Geometry: final body of the model. Coordinates: model frame, mm. A direction names the side the tool comes from. Give positions to 0.01 mm unless a question says otherwise; leave off trailing zeros. Write each loop counter-clockwise with the first axis right and the second up, starting at its lowest first coordinate (ties: lowest second). Pieces come first, ordered by that corner, then holes. Notation, with made-up numbers: (30.5, 53.25) -> (63.5, 53.25) arc R15 cw to (63.5, 73.25) -> close; hole circle Ø7 at (30.25, 85). An arc over 180 degrees is marked (long way). Use CSV: the item, a comma, the result in double quotes. Start each with the question number.
1) Material intervals for line 1 (Z direction, x = -9.5, y = -1.7); line 2 (X direction, y = 0.25, z = -103.5); line 3 (X direction, y = -1.7, z = -16.75), sorted ascending. Write a range as [from, to].
2) Set-up query: faces 4 (the face through (9, 0, 0)), 5 (the face through (36.5, 1, -25)), 6 (the face through (88, 0, -46)). Return all of +Z, -Z, +X, -X, +Y, -Y with unobstructed straight access to the full face (end or side cutting, diameter ignored); none if empty.
3) Section A-A (x = 76.5). Output: boundary loops of the cut face in (y, z).
4) Draft query along X for faces 1 (the face through (12, -0.5, -7.3)), 2 (the face through (17.9, -3.5, -74.6)), 3 (the face through (15, 0, -68)). Return one class per face: pulls with the +X half, pulls with the -X half, needs draft (parallel to the pull), parting line crosses it, or undercut.
5) Section B-B (y = -1.45). Count the separate pieces of the cut face and the enclosed holes in it, plus the area to 3 significant figures.
6) Contact query for flat-ended pins moving along their axis: P1, Ø1.8, axis at x = 41, y = -2.5, coming from the -Z side; P2, Ø0.8, axis at y = 0.5, z = -1.5, coming from the -X side; P3, Ø2.5, axis at x = 34, y = -2.5, coming from the +Z side. Output: stop coordinate, or through.
```python
from build123d import *

# Parameters (mm, degrees)
SKETCH2_W                      = 14
SKETCH2_H                      = 14
BOSS_EXTRUDE1_DEPTH            = 1.5
SKETCH3_R                      = 7.5
SKETCH3_R_2                    = 4.250000483
SKETCH3_R_3                    = 4.259363822
SKETCH3_W                      = 5
SKETCH3_H                      = 5
SKETCH3_W_2                    = 29.940596835
SKETCH3_W_3                    = 6
SKETCH3_W_4                    = 15
SKETCH3_H_2                    = 15
SKETCH3_W_5                    = 2.885686077
SKETCH3_H_3                    = 6.92
SKETCH3_W_6                    = 48.043350903
SKETCH3_H_4                    = 3
BOSS_EXTRUDE2_DEPTH            = 3.5
M3_CLEARANCE_HOLE1_D           = 3.6
M3_CLEARANCE_HOLE1_CSINK_D     = 3.65
M3_CLEARANCE_HOLE1_CSINK_ANGLE = 90


with BuildPart() as part:
    # Sketch2 → Boss-Extrude1 (new body)
    with BuildSketch(Plane(origin=(0, 0, 0), x_dir=(1, 0, 0), z_dir=(0, 1, 0))):
        Polygon((90.5, 34), (90.5, 88.92), (105.066, 88.92), (105.066, 112.92), (34.566, 112.92), (34.566, 101.999439424), (12.680313923, 101.999439424), (12.680313923, 95.731483365), (-40.408317869, 95.731483365), (-44.678770934, 85.421697657), (-65.29834235, 85.421697657), (-69.197497471, 76.008304483), (-102.403943224, 76.008304483), (-102.403943224, 52.008304483), (-53.463346389, 52.008304483), (-12, 34.833624067), (-12, -12), (12, -12), (12, 20), (36.5, 20), (36.5, 34), align=None)
        with Locations((-90.403943224, 64.008304483)):
            Rectangle(SKETCH2_W, SKETCH2_H, mode=Mode.SUBTRACT)
        Polygon((-67.315017213, 67.487384202), (-61.95744916, 80.421697657), (-49.023135705, 75.064129604), (-54.380703758, 62.129816149), align=None, mode=Mode.SUBTRACT)
        with Locations((46.566, 100.92)):
            Rectangle(SKETCH2_W, SKETCH2_H, mode=Mode.SUBTRACT)
        Polygon((-31.423230611, 67.774010218), (-44.357544066, 73.131578271), (-49.715112119, 60.197264816), (-36.780798664, 54.839696762), align=None, mode=Mode.SUBTRACT)
        with Locations((-0.524094275, 75.65587615)):
            Rectangle(SKETCH2_W, SKETCH2_H, mode=Mode.SUBTRACT)
        with Locations((24.680313923, 89.999439424)):
            Rectangle(SKETCH2_W, SKETCH2_H, mode=Mode.SUBTRACT)
        with Locations((24.5, 61)):
            Rectangle(SKETCH2_W, SKETCH2_H, mode=Mode.SUBTRACT)
        with Locations((24.5, 32)):
            Rectangle(SKETCH2_W, SKETCH2_H, mode=Mode.SUBTRACT)
        with Locations((49.5, 46)):
            Rectangle(SKETCH2_W, SKETCH2_H, mode=Mode.SUBTRACT)
        with Locations((49.5, 75)):
            Rectangle(SKETCH2_W, SKETCH2_H, mode=Mode.SUBTRACT)
        with Locations((78.5, 75)):
            Rectangle(SKETCH2_W, SKETCH2_H, mode=Mode.SUBTRACT)
        with Locations((78.5, 46)):
            Rectangle(SKETCH2_W, SKETCH2_H, mode=Mode.SUBTRACT)
        Rectangle(SKETCH2_W, SKETCH2_H, mode=Mode.SUBTRACT)
        Polygon((-33.645940754, 49.211627299), (-20.711627299, 43.854059246), (-15.354059246, 56.788372701), (-28.288372701, 62.145940754), align=None, mode=Mode.SUBTRACT)
        Polygon((-42.424992732, 77.79716991), (-37.067424679, 90.731483365), (-24.133111224, 85.373915312), (-29.490679277, 72.439601857), align=None, mode=Mode.SUBTRACT)
        with Locations((62.066, 100.92)):
            Rectangle(SKETCH2_W, SKETCH2_H, mode=Mode.SUBTRACT)
        with Locations((77.566, 100.92)):
            Rectangle(SKETCH2_W, SKETCH2_H, mode=Mode.SUBTRACT)
        with Locations((93.066, 100.92)):
            Rectangle(SKETCH2_W, SKETCH2_H, mode=Mode.SUBTRACT)
    extrude(amount=BOSS_EXTRUDE1_DEPTH)

    # Sketch3 → Boss-Extrude2 (add)
    with BuildSketch(Plane.XZ):
        with Locations(Location((-0.403943224, -53.000000483, 0), (0, 0, 90))):
            Circle(SKETCH3_R)
        with Locations(Location((-0.903943224, -16.750000483, 0), (0, 0, 90))):
            Circle(SKETCH3_R_2)
        with Locations(Location((41.096056776, -60.500000483, 0), (0, 0, 90))):
            Circle(SKETCH3_R_3)
        with Locations(Location((16.096056776, -75.500000483, 0), (0, 0, 90))):
            Circle(SKETCH3_R_3)
        Polygon((-20.711627299, -43.854059246), (-22.625044461, -39.234661583), (-12, -34.833624067), (-12, -7), (-7, -7), (-7, -40.245585068), (-12, -40.245585068), align=None)
        with Locations((37.066, -110.42)):
            Rectangle(SKETCH3_W, SKETCH3_H)
        with Locations((102.566, -110.42)):
            Rectangle(SKETCH3_W, SKETCH3_H)
        with Locations((102.566, -91.42)):
            Rectangle(SKETCH3_W, SKETCH3_H)
        with Locations((88, -36.5)):
            Rectangle(SKETCH3_W, SKETCH3_H)
        with Locations((34, -22.5)):
            Rectangle(SKETCH3_W, SKETCH3_H)
        with Locations((9.5, 9.5)):
            Rectangle(SKETCH3_W, SKETCH3_H)
        with Locations((-9.5, 9.5)):
            Rectangle(SKETCH3_W, SKETCH3_H)
        with Locations((-99.903943224, -54.508304483)):
            Rectangle(SKETCH3_W, SKETCH3_H)
        with Locations((-99.903943224, -73.508304483)):
            Rectangle(SKETCH3_W, SKETCH3_H)
        Polygon((17.5, -25), (7, -25), (7, -7), (12, -7), (12, -20), (17.5, -20), align=None)
        with Locations((-68.433644806, -54.508304483)):
            Rectangle(SKETCH3_W_2, SKETCH3_H)
        with Locations((15.180313923, -99.499439424)):
            Rectangle(SKETCH3_W, SKETCH3_H)
        with BuildLine():
            Line((-83.403943224, -71.008304483), (-76.205169586, -71.008304483))
            ThreePointArc((-76.205169586, -71.008304483), (-70.746354877, -68.438373932), (-69.197497471, -74.269689546))
            Line((-69.197497471, -74.269689546), (-69.197497471, -76.008304483))
            Line((-69.197497471, -76.008304483), (-83.403943224, -76.008304483))
            Line((-83.403943224, -76.008304483), (-83.403943224, -71.008304483))
        make_face()
        with Locations((39.5, -36.5)):
            Rectangle(SKETCH3_W_3, SKETCH3_H)
        with Locations((64, -36.5)):
            Rectangle(SKETCH3_W_4, SKETCH3_H)
        with Locations((88, -60.5)):
            Rectangle(SKETCH3_W, SKETCH3_H_2)
        with Locations((33.123156962, -99.499439424)):
            Rectangle(SKETCH3_W_5, SKETCH3_H)
        with Locations((88, -85.46)):
            Rectangle(SKETCH3_W, SKETCH3_H_3)
        with Locations((-11.341361529, -94.231483365)):
            Rectangle(SKETCH3_W_6, SKETCH3_H_4)
    extrude(amount=BOSS_EXTRUDE2_DEPTH)

    # M3 Clearance Hole1 (through all)
    with Locations(Plane(origin=(-0.403943224, -3.5, -53.000000483), x_dir=(0, 0, -1), z_dir=(0, -1, 0))):
        with Locations((0, 0), (7.5, 41.5), (22.5, 16.5), (-36.25, -0.5), (19, -72)):
            CounterSinkHole(M3_CLEARANCE_HOLE1_D / 2, M3_CLEARANCE_HOLE1_CSINK_D / 2, counter_sink_angle=M3_CLEARANCE_HOLE1_CSINK_ANGLE)


solid = part.part
```
Answers follow:
1,line 1,"z = [-95.73, -92.73], [-40.25, -7], [7, 12]"
1,line 2,"x = [34.57, 39.57], [53.57, 55.07], [69.07, 70.57], [84.57, 86.07], [100.07, 105.07]"
1,line 3,"x = [-12, -7], [-5.15, -2.7], [0.9, 3.35], [7, 12]"
2,face 4,"+X, -X, -Y"
2,face 5,"+Z, +X, +Y, -Y"
2,face 6,"+X, -Y"
3,outline,"(0, -112.92) -> (1.5, -112.92) -> (1.5, -107.92) -> (0, -107.92) -> close; (0, -93.92) -> (1.5, -93.92) -> (1.5, -82) -> (0, -82) -> close; (0, -68) -> (1.5, -68) -> (1.5, -53) -> (0, -53) -> close; (0, -39) -> (1.5, -39) -> (1.5, -34) -> (0, -34) -> close"
4,face 1,"pulls with the +X half"
4,face 2,"needs draft"
4,face 3,"undercut"
5,separate pieces,"24"
5,enclosed holes,"5"
5,area,"1,490 mm^2"
6,P1,"stops at z = -64.76"
6,P2,"stops at x = -12"
6,P3,"stops at z = -20"
